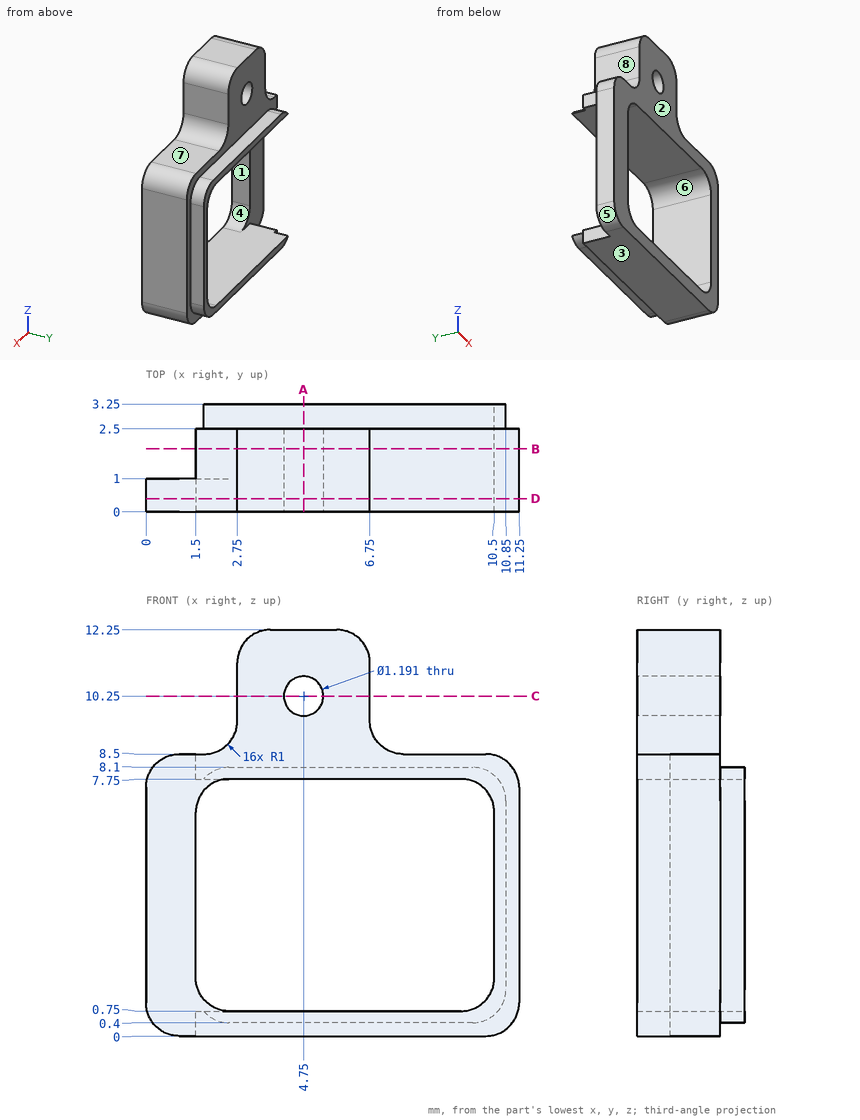
The figure shows three views and two pictorial views of one solid part (mm, origin at its lowest corner). Answer the questions. A direction names the side the tool comes from. Give positions to 0.01 mm unless a question says otherwise; leave off trailing zeros. Write each loop counter-clockwise with the first axis right and the second up, starting at its lowest first coordinate (ties: lowest second). Pieces come first, ordered by that corner, then holes. Notation, with made-up numbers: (23.25, 11) - (46.25, 11) arc R24 ccw to (46.25, 35) - close; hole circle Ø9 at (15, 64.25). An arc over 180 degrees is marked (long way). Return JSON: item names as keys, results as strings.
Q1. Given P1, Ø1.9, axis at x = 4.75, z = 10.25, coming from the -Y side; P2, Ø1, axis at y = 3, z = 2.5, coming from the -X side; P3, Ø1.4, axis at y = 1.5, z = 10, coming from the +X side; P4, Ø0.5, axis at y = 1.5, z = 10.5, coming from the -X side, each flat-ended and moving along its own axis, determine where each tip first touches the part or whether it passes through.
Reply:
{"P1": "y = 0", "P2": "x = 10.5", "P3": "x = 6.77", "P4": "x = 2.75"}
Q2. For a pull along Z with two mould halves and no side action, classify the marked faces 1, 2, 3 and 4 as released by +Z, released by -Z, zero draft, split by the parting line, or undercut.
Reply:
{"face 1": "undercut", "face 2": "zero draft", "face 3": "released by -Z", "face 4": "undercut"}
Q3. For the marked faces 5, 6, 7 and 8, determine the directions among +Z, -Z, +X, -X, +Y, -Y from which every point of the face is accessible in a straight line to the end or side of a thin tool.
Reply:
{"face 5": "-Z, -X, +Y, -Y", "face 6": "+Y, -Y", "face 7": "+Z, +X, +Y, -Y", "face 8": "+Z, -X, +Y, -Y"}
Q4. Consider line 1 along X through (y, z) = (1, 10.25); line 2 along Z through (x, y) = (9.25, 1.8); line 3 along X through (y, z) = (0.2, 3). Determine where each line is inside the solid, lowest interval first. Write a range as [from, to].
Reply:
{"line 1": "[2.75, 4.15], [5.35, 6.75]", "line 2": "[0, 0.75], [7.75, 8.5]", "line 3": "[0, 1.5], [10.5, 11.25]"}
Q5. A cutting plane is placed at D-D, the plane y = 0.4. Determine the outline of the cut face in (x, z).
Reply:
{"outline": "(0, 1) arc R1 ccw to (1, 0) - (10.25, 0) arc R1 ccw to (11.25, 1) - (11.25, 7.5) arc R1 ccw to (10.25, 8.5) - (7.75, 8.5) arc R1 cw to (6.75, 9.5) - (6.75, 11.25) arc R1 ccw to (5.75, 12.25) - (3.75, 12.25) arc R1 ccw to (2.75, 11.25) - (2.75, 9.5) arc R1 cw to (1.75, 8.5) - (1, 8.5) arc R1 ccw to (0, 7.5) - close; hole (1.5, 1.75) arc R1 ccw to (2.5, 0.75) - (9.5, 0.75) arc R1 ccw to (10.5, 1.75) - (10.5, 6.75) arc R1 ccw to (9.5, 7.75) - (2.5, 7.75) arc R1 ccw to (1.5, 6.75) - close; hole circle Ø1.19 at (4.75, 10.25)"}
Q6. A cutting plane is placed at B-B, the plane y = 1.9. Determine the outline of the cut face in (x, z).
Reply:
{"outline": "(1.5, 0) - (10.25, 0) arc R1 ccw to (11.25, 1) - (11.25, 7.5) arc R1 ccw to (10.25, 8.5) - (7.75, 8.5) arc R1 cw to (6.75, 9.5) - (6.75, 11.25) arc R1 ccw to (5.75, 12.25) - (3.75, 12.25) arc R1 ccw to (2.75, 11.25) - (2.75, 9.5) arc R1 cw to (1.75, 8.5) - (1.5, 8.5) - (1.5, 7.75) - (9.5, 7.75) arc R1 cw to (10.5, 6.75) - (10.5, 1.75) arc R1 cw to (9.5, 0.75) - (1.5, 0.75) - close; hole circle Ø1.19 at (4.75, 10.25)"}
Q7. A cutting plane is placed at A-A, the plane x = 4.75. Determine the outline of the cut face in (y, z).
Reply:
{"outline": "(0, 0) - (2.5, 0) - (2.5, 0.4) - (3.25, 0.4) - (3.25, 0.75) - (0, 0.75) - close; (0, 7.75) - (3.25, 7.75) - (3.25, 8.1) - (2.5, 8.1) - (2.5, 9.65) - (0, 9.65) - close; (0, 10.85) - (2.5, 10.85) - (2.5, 12.25) - (0, 12.25) - close"}
Q8. A cutting plane is placed at C-C, the plane z = 10.25. Determine the outline of the cut face in (x, y).
Reply:
{"outline": "(2.75, 0) - (4.15, 0) - (4.15, 2.5) - (2.75, 2.5) - close; (5.35, 0) - (6.75, 0) - (6.75, 2.5) - (5.35, 2.5) - close"}
